from build123d import *

# Parameters (mm, degrees)
FILLET1_R = 0.5
SKETCH4_R = 0.3


with BuildPart() as part:
    # Sketch1 → Revolve1 (revolve)
    with BuildSketch(Plane.XY, mode=Mode.PRIVATE) as revolve1_sk:
        Polygon((0, 0), (3.25, 0), (3.25, 0.3), (2.75, 1.25), (1.75, 1.25), (1.25, 0.986842105), (-1.25, 0.986842105), (-1.75, 1.25), (-2.75, 1.25), (-3.25, 0.3), (-3.25, 0), align=None)
    revolve(revolve1_sk.sketch.rotate(Axis((0, 0, 0), (1, 0, 0)), 90), axis=Axis((0, 0, 0), (1, 0, 0)))

    # Fillet1
    fillet1_edges = [part.edges().sort_by_distance(p)[0] for p in [
        (1.75, 0, -1.25),
        (2.75, 0, -1.25),
        (-2.75, 0, -1.25),
        (-1.75, 0, -1.25),
        (-1.25, 0, -0.986842105),
        (1.25, 0, -0.986842105),
    ]]
    fillet(fillet1_edges, radius=FILLET1_R)

    # Sweep1: sweep along a path in Sketch6
    with BuildLine(Plane.XY) as sweep1_path:
        Line((5.08, 3), (5.08, 0.75))
        ThreePointArc((5.08, 0.75), (4.860330086, 0.219669914), (4.33, 0))
        Line((4.33, 0), (3.25, 0))
        Line((3.25, 0), (-4.33, 0))
        ThreePointArc((-4.33, 0), (-4.860330086, 0.219669914), (-5.08, 0.75))
        Line((-5.08, 0.75), (-5.08, 3))
    # Sketch4 → Sweep1 (sweep)
    with BuildSketch(Plane(origin=(3.25, 0, 0), x_dir=(0, 0, -1), z_dir=(1, 0, 0))):
        Circle(SKETCH4_R)
    sweep(path=sweep1_path.line)


solid = part.part
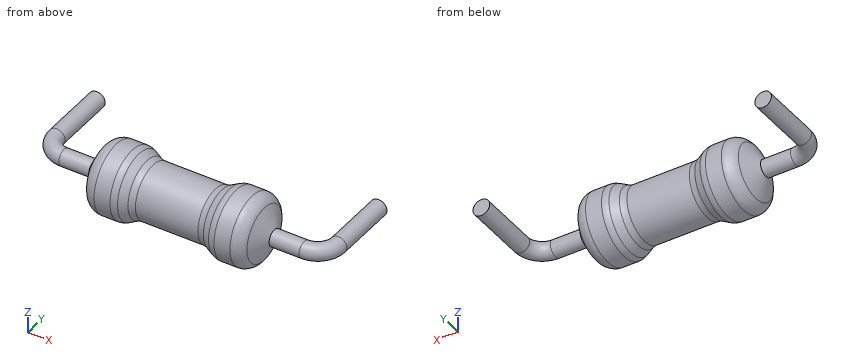
Work out the finished part from the listing and answer in its coordinate system (mm). Give positions to 0.01 mm unless a question says otherwise; leave off trailing zeros. Loops run counter-clockwise (first coordinate to the right, second up) from the corner with the lowest first, then second, coordinate; pieces in that order, holes last. Notation, with made-up numbers: (33.5, 4) -> (43.5, 4) arc R7 cw to (43.5, 10) -> close; hole circle Ø1 at (34, 0.5). An arc over 180 degrees is marked (long way). Use a Markdown table: item, result. Add a question column.
1) The part is cut by section B-B, the plane x = -4. Determine the outline of the cut face in (y, z), plus the area to 3 significant figures.
2) This flat-tipped pin is pushed along its axis until it touches: P1, Ø1, axis at y = 0.5, z = -0.5, coming from the -X side. Where does it stop, or does it pass through?
3) The part is cut by section A-A, the plane y = 2.1. Determine the outline of the cut face in (x, z), plus the area to 3 significant figures.
4) Consider line 1 along Y through (x, z) = (1.5, 0.4); line 2 along X through (y, z) = (1.1, 0) (3 decimals); line 3 along Z through (x, y) = (-4.75, 0.1). Determine where each line is inside the solid, lowest interval first.
5) The part is cut by section C-C, the plane x = -1. Determine the outline of the cut face in (y, z), plus the area to 3 significant figures.
Reported:
| question | item | result |
|---|---|---|
| 1 | outline | circle Ø0.6 at (0, 0) |
| 1 | area | 0.283 mm^2 |
| 2 | P1 | stops at x = -5.38 |
| 3 | outline | circle Ø0.6 at (-5.08, 0); circle Ø0.6 at (5.08, 0) |
| 3 | area | 0.565 mm^2 |
| 4 | line 1 | y = -1.04 to 1.04 |
| 4 | line 2 | x = -5.38 to -4.78, -2.805 to -1.465, 1.465 to 2.805, 4.78 to 5.38 |
| 4 | line 3 | z = -0.3 to 0.3 |
| 5 | outline | circle Ø1.97 at (0, 0) |
| 5 | area | 3.06 mm^2 |
